from build123d import *

# Parameters (mm, degrees)
SKETCH1_R           = 250
BOSS_EXTRUDE1_DEPTH = 65
CHAMFER1_SIZE       = 20
SKETCH2_R           = 190
CUT_EXTRUDE1_DEPTH  = 20
CUT_EXTRUDE1_TAPER  = 45
SKETCH3_R           = 190
CUT_EXTRUDE2_DEPTH  = 20
CUT_EXTRUDE2_TAPER  = 45
SKETCH4_R           = 31
SKETCH4_R_2         = 39
CUT_EXTRUDE3_DEPTH  = 111.0000001


with BuildPart() as part:
    # Sketch1 → Boss-Extrude1 (new body, symmetric)
    with BuildSketch(Plane.XY):
        Circle(SKETCH1_R)
    extrude(amount=BOSS_EXTRUDE1_DEPTH, both=True)

    # Chamfer1
    chamfer1_edges = [part.edges().sort_by_distance(p)[0] for p in [
        (-250, 0, -65),
        (-250, 0, 65),
    ]]
    chamfer(chamfer1_edges, length=CHAMFER1_SIZE)

    # Sketch2 → Cut-Extrude1 (cut)
    with BuildSketch(Plane.XY.offset(65)):
        Circle(SKETCH2_R)
    extrude(amount=-CUT_EXTRUDE1_DEPTH, taper=CUT_EXTRUDE1_TAPER, mode=Mode.SUBTRACT)

    # Sketch3 → Cut-Extrude2 (cut)
    with BuildSketch(Plane(origin=(0, 0, -65), x_dir=(-1, 0, 0), z_dir=(0, 0, -1))):
        Circle(SKETCH3_R)
    extrude(amount=-CUT_EXTRUDE2_DEPTH, taper=CUT_EXTRUDE2_TAPER, mode=Mode.SUBTRACT)

    # Sketch4 → Cut-Extrude3 (cut, through all)
    with BuildSketch(Plane(origin=(0, 0, -45), x_dir=(-1, 0, 0), z_dir=(0, 0, -1))):
        with Locations((0, 100)):
            Circle(SKETCH4_R)
        with Locations((-100, 0)):
            Circle(SKETCH4_R)
        with Locations((0, -100)):
            Circle(SKETCH4_R)
        with Locations((100, 0)):
            Circle(SKETCH4_R)
        Circle(SKETCH4_R_2)
    extrude(amount=-CUT_EXTRUDE3_DEPTH, mode=Mode.SUBTRACT)


solid = part.part
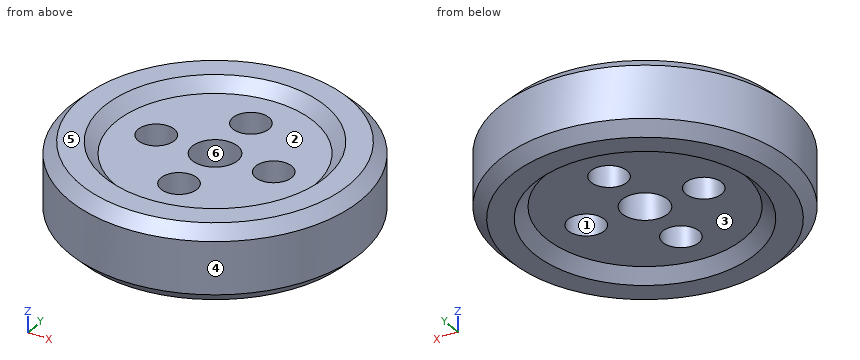
Design review of the part built by this model. Coordinates are the model's own, in mm. Face numbers are marked on the shaded views. A direction names the side the tool comes from. Coordinates: 2 decimals unless noted, no trailing zeros. Loops run counter-clockwise (first coordinate to the right, second up) from the corner with the lowest first, then second, coordinate; pieces in that order, holes last. Notation, with made-up numbers: (54.25, 16.5) -> (110.25, 16.5) arc R10 cw to (110.25, 34.5) -> close; hole circle Ø10 at (84.5, 23). An arc over 180 degrees is marked (long way). Use a Markdown table: item, result. Add a question column.
Item 1: We need section C-C, the plane y = 0. Count the separate pieces of the cut face and the enclosed holes in it, and give its area (3 significant figures).
Item 2: We need section B-B, the plane z = 29. Write out the cut boundary in (x, y), and give its area (3 significant figures).
Item 3: The part is to be moulded in two halves that separate along X. For the marked faces 4, 5 and 6, say which applies: +X half, -X half, draft (parallel to the pull), parting line (faces both ways), or undercut.
Item 4: Wall thickness on L1, parallel to Y at x = 0, z = -2; L2, parallel to X at y = 2, z = -30; L3, parallel to X at y = 13, z = -42: over which ranges is each line inside the solid? List them lowest first. Write a range as from..to.
Item 5: Machinability: for the marked faces 1, 2 and 3, which of the approach directions +Z, -Z, +X, -X, +Y, -Y give a long, thin tool a straight path to every point of the face, cutting with its end or side? Answer none if there is none.
Item 6: Clearance check with flat-ended pins moving along their axes: P1, Ø8, axis at y = 37, z = 46.5, coming from the +X side; P2, Ø1.5, axis at y = 23, z = -25, coming from the +X side; P3, Ø6, axis at y = -126.5, z = -24.5, coming from the +X side. State where each tip first meets the part, or that it passes through.
Item 7: We need section A-A, the plane x = 0. Write out the cut boundary in (y, z), and give its area (3 significant figures).
Item 8: We need section D-D, the plane z = -52.5. Write out the cut boundary in (x, y).
Numbers:
| question | item | result |
|---|---|---|
| 1 | separate pieces | 4 |
| 1 | enclosed holes | 0 |
| 1 | area | 31,600 mm^2 |
| 2 | outline | circle Ø500 at (0, 0); hole circle Ø62 at (-100, 0); hole circle Ø78 at (0, 0); hole circle Ø62 at (0, -100); hole circle Ø62 at (0, 100); hole circle Ø62 at (100, 0) |
| 2 | area | 179,000 mm^2 |
| 3 | face 4 | parting line |
| 3 | face 5 | draft |
| 3 | face 6 | undercut |
| 4 | L1 | y = -250..-131, -69..-39, 39..69, 131..250 |
| 4 | L2 | x = -249.99..-130.94, -69.06..-38.95, 38.95..69.06, 130.94..249.99 |
| 4 | L3 | x = -249.66..-128.14, -71.86..-36.77, 36.77..71.86, 128.14..249.66 |
| 5 | face 1 | +Z, -Z |
| 5 | face 2 | +Z |
| 5 | face 3 | -Z |
| 6 | P1 | stops at x = 247.77 |
| 6 | P2 | stops at x = 249.01 |
| 6 | P3 | stops at x = 217.37 |
| 7 | outline | (-250, -45) -> (-230, -65) -> (-190, -65) -> (-170, -45) -> (-131, -45) -> (-131, 45) -> (-170, 45) -> (-190, 65) -> (-230, 65) -> (-250, 45) -> close; (-69, -45) -> (-39, -45) -> (-39, 45) -> (-69, 45) -> close; (39, -45) -> (69, -45) -> (69, 45) -> (39, 45) -> close; (131, -45) -> (170, -45) -> (190, -65) -> (230, -65) -> (250, -45) -> (250, 45) -> (230, 65) -> (190, 65) -> (170, 45) -> (131, 45) -> close |
| 7 | area | 31,600 mm^2 |
| 8 | outline | circle Ø485 at (0, 0); hole circle Ø355 at (0, 0) |
